Here's how the part is built. I have some questions about the finished solid (model axes, mm). Face numbers are marked on the shaded views. Round coordinates to 2 decimals unless told otherwise and drop trailing zeros. Loops run counter-clockwise (first coordinate to the right, second up) from the corner with the lowest first, then second, coordinate; pieces in that order, holes last. Notation, with made-up numbers: (5, -29.5) -> (52, -29.5) arc R29 cw to (52, -6.5) -> close; hole circle Ø11 at (6, 43). An arc over 180 degrees is marked (long way). One line per item, written item: value. Start each with the question number.
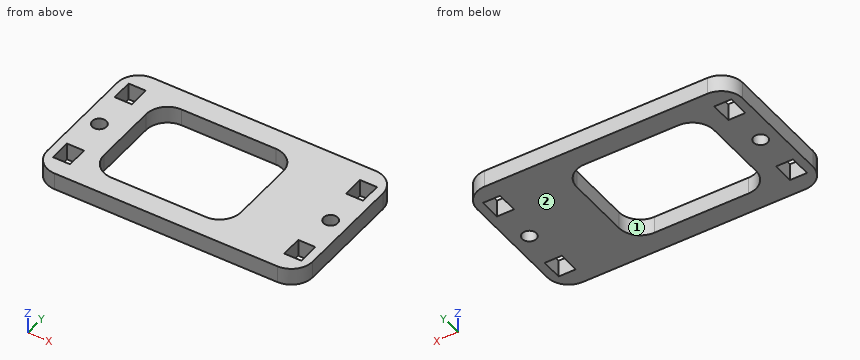
```python
from build123d import *

# Parameters (mm, degrees)
F0_W     = 62
F0_H     = 35
F0_W_2   = 4
F0_H_2   = 5
F0_W_3   = 32
F0_H_3   = 25
F1_DEPTH = 4
F2_D     = 3.3
F3_R     = 5
F4_R     = 5


with BuildPart() as f1:
    # F0 (on Top) → F1 (new body)
    with BuildSketch(Plane.XY):
        Rectangle(F0_W, F0_H)
        with Locations((-27, -11)):
            Rectangle(F0_W_2, F0_H_2, mode=Mode.SUBTRACT)
        with Locations((27, -11)):
            Rectangle(F0_W_2, F0_H_2, mode=Mode.SUBTRACT)
        with Locations((-5, 0)):
            Rectangle(F0_W_3, F0_H_3, mode=Mode.SUBTRACT)
        with Locations((-27, 11)):
            Rectangle(F0_W_2, F0_H_2, mode=Mode.SUBTRACT)
        with Locations((27, 11)):
            Rectangle(F0_W_2, F0_H_2, mode=Mode.SUBTRACT)
    extrude(amount=F1_DEPTH)

    # F2 (through all)
    with Locations(Plane(origin=(0, 0, 0), x_dir=(1, 0, 0), z_dir=(0, 0, -1))):
        with Locations((-27, 0), (27, 0)):
            Hole(F2_D / 2)

    # F3
    f3_edges = [f1.edges().sort_by_distance(p)[0] for p in [
        (-31, -17.5, 2),
        (31, -17.5, 2),
        (31, 17.5, 2),
        (-31, 17.5, 2),
    ]]
    fillet(f3_edges, radius=F3_R)

    # F4
    f4_edges = [f1.edges().sort_by_distance(p)[0] for p in [
        (-21, 12.5, 2),
        (11, 12.5, 2),
        (11, -12.5, 2),
        (-21, -12.5, 2),
    ]]
    fillet(f4_edges, radius=F4_R)


solid = f1.part
```
Q1. I want a section at C-C on y = 0. Please give me the cut outline in (x, z).
Q2. I want a section at A-A on z = 1.1. State how many separate pieces and enclosed holes the cut face has, plus the area to 3 significant figures.
Q3. Will these pins go through, and if not, where does the flat tip stop? P1, Ø10, axis at x = 2.5, y = 2.5, coming from the -Z side; P2, Ø1.2, axis at x = -28, z = 2, coming from the +Y side.
Q4. If I drill on line 1 along Y through (x, z) = (-2.5, 3.35); line 2 along X through (y, z) = (-9, 2.8); line 3 along Y through (x, z) = (-27, 1.4), over which ranges is the centre line in solid material (lowest first)?
Q5. I want a section at B-B on x = 3. Please give me the cut outline in (y, z), plus the area to 3 significant figures.
Q6. I want a section at D-D on y = -6. Please give me the cut outline in (x, z).
Q7. If we mould it in two halves opening along Y, with no side actions, what happens to the marked faces 1 and 2? For each: released by +Y, released by -Y, zero draft, split by the parting line, or undercut.
Answers below:
1. outline: (-31, 0) -> (-28.65, 0) -> (-28.65, 4) -> (-31, 4) -> close; (-25.35, 0) -> (-21, 0) -> (-21, 4) -> (-25.35, 4) -> close; (11, 0) -> (25.35, 0) -> (25.35, 4) -> (11, 4) -> close; (28.65, 0) -> (31, 0) -> (31, 4) -> (28.65, 4) -> close
2. separate pieces: 1
2. enclosed holes: 7
2. area: 1,270 mm^2
3. P1: passes through
3. P2: stops at y = 17.3
4. line 1: y = -17.5 to -12.5, 12.5 to 17.5
4. line 2: x = -31 to -29, -25 to -20.77, 10.77 to 25, 29 to 31
4. line 3: y = -17.4 to -13.5, -8.5 to -1.65, 1.65 to 8.5, 13.5 to 17.4
5. outline: (-17.5, 0) -> (-12.5, 0) -> (-12.5, 4) -> (-17.5, 4) -> close; (12.5, 0) -> (17.5, 0) -> (17.5, 4) -> (12.5, 4) -> close
5. area: 40.0 mm^2
6. outline: (-31, 0) -> (-21, 0) -> (-21, 4) -> (-31, 4) -> close; (11, 0) -> (31, 0) -> (31, 4) -> (11, 4) -> close
7. face 1: undercut
7. face 2: zero draft
